```python
from build123d import *

# Parameters (mm, degrees)
SKETCH_1_R          = 3.5
EXTRUDE_1_DEPTH     = 4
SKETCH_3_R          = 3.5
EXTRUDE_2_DEPTH     = 2.9
SKETCH_4_W          = 4.5
SKETCH_4_H          = 4.5
EXTRUDE_3_DEPTH     = 2.5
SKETCH_7_R          = 3.5
CUT_EXTRUDE_1_DEPTH = 10


with BuildPart() as part:
    # 草图1 → 凸台-拉伸1 (new body)
    with BuildSketch(Plane(origin=(0, 0, 0), x_dir=(1, 0, 0), z_dir=(0, 1, 0))):
        Circle(SKETCH_1_R)
        with BuildLine():
            Line((-2.25, 2.25), (-0.4, 2.25))
            ThreePointArc((-0.4, 2.25), (0, 2.65), (0.4, 2.25))
            Line((0.4, 2.25), (2.25, 2.25))
            Line((2.25, 2.25), (2.25, 0.4))
            ThreePointArc((2.25, 0.4), (2.65, 0), (2.25, -0.4))
            Line((2.25, -0.4), (2.25, -2.25))
            Line((2.25, -2.25), (0.4, -2.25))
            ThreePointArc((0.4, -2.25), (0, -2.65), (-0.4, -2.25))
            Line((-0.4, -2.25), (-2.25, -2.25))
            Line((-2.25, -2.25), (-2.25, -0.4))
            ThreePointArc((-2.25, -0.4), (-2.65, 0), (-2.25, 0.4))
            Line((-2.25, 0.4), (-2.25, 2.25))
        make_face(mode=Mode.SUBTRACT)
    extrude(amount=EXTRUDE_1_DEPTH)

    # 草图3 → 凸台-拉伸2 (add)
    with BuildSketch(Plane(origin=(0, 4, 0), x_dir=(1, 0, 0), z_dir=(0, 1, 0))):
        Circle(SKETCH_3_R)
    extrude(amount=EXTRUDE_2_DEPTH)

    # 草图4 → 凸台-拉伸3 (add)
    with BuildSketch(Plane(origin=(0, 6.9, 0), x_dir=(1, 0, 0), z_dir=(0, 1, 0))):
        Rectangle(SKETCH_4_W, SKETCH_4_H)
    extrude(amount=EXTRUDE_3_DEPTH)

    # 草图5 → 旋转1 (revolve)
    with BuildSketch(Plane(origin=(0, 9.4, 0), x_dir=(1, 0, 0), z_dir=(0, 1, 0))):
        with BuildLine():
            Line((-2.75, 0), (-1.75, 0))
            ThreePointArc((-1.75, 0), (-2.25, -0.5), (-2.75, 0))
        make_face()
        with BuildLine():
            Line((1.75, 0), (2.75, 0))
            ThreePointArc((2.75, 0), (2.25, -0.5), (1.75, 0))
        make_face()
    revolve(axis=Axis((-2.75, 9.4, 0), (1, 0, 0)))

    # 草图6 → 旋转2 (revolve)
    with BuildSketch(Plane(origin=(0, 9.4, 0), x_dir=(1, 0, 0), z_dir=(0, 1, 0))):
        with BuildLine():
            Line((0, -2.75), (0, -1.75))
            ThreePointArc((0, -1.75), (-0.5, -2.25), (0, -2.75))
        make_face()
        with BuildLine():
            Line((0, 1.75), (0, 2.75))
            ThreePointArc((0, 2.75), (-0.5, 2.25), (0, 1.75))
        make_face()
    revolve(axis=Axis((0, 9.4, 2.75), (0, 0, -1)))

    # 草图7 → 切除-拉伸1 (cut)
    with BuildSketch(Plane(origin=(0, 9.4, 0), x_dir=(1, 0, 0), z_dir=(0, 1, 0))):
        Circle(SKETCH_7_R)
    extrude(amount=CUT_EXTRUDE_1_DEPTH, mode=Mode.SUBTRACT)


solid = part.part
```
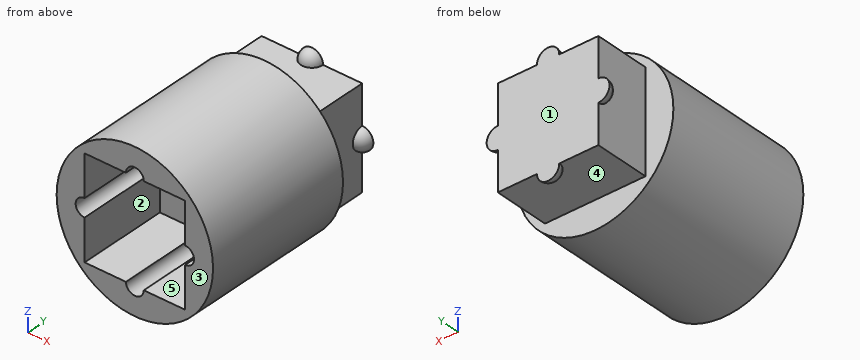
Verification items for the finished model (mm, model axes). Face numbers are marked on the shaded views. A direction names the side the tool comes from. Give positions to 0.01 mm unless a question says otherwise; leave off trailing zeros. Loops run counter-clockwise (first coordinate to the right, second up) from the corner with the lowest first, then second, coordinate; pieces in that order, holes last. Notation, with made-up numbers: M 56,38 L 110,38 A38 cw 110,77 Z; hole C 6,36 d10. An arc over 180 degrees is marked long. Return JSON: item names as keys, results as strings.
1) Gauge pin test, flat ends, axial feed: P1, Ø1, axis at y = 8, z = -1.5, coming from the +X side; P2, Ø1.5, axis at y = 2, z = 1, coming from the +X side; P3, Ø0.6, axis at y = 2.5, z = -1, coming from the -X side. Record the tip position at first contact, or that the pin passes through.
Findings:
{"P1": "stops at x = 2.25", "P2": "stops at x = 3.49", "P3": "stops at x = -3.43"}
2) Section check C-C, the plane x = 0. Enter the section's corners in (y, z).
Findings:
{"outline": "M 0,-3.5 L 6.9,-3.5 L 6.9,-2.25 L 8.9,-2.25 A0.5 ccw 9.4,-2.75 L 9.4,2.75 A0.5 ccw 8.9,2.25 L 6.9,2.25 L 6.9,3.5 L 0,3.5 L 0,2.65 L 4,2.65 L 4,-2.65 L 0,-2.65 Z"}
3) Section check D-D, the plane y = 8. Enter the section's corners in (x, z), and give its area (4 significant figures).
Findings:
{"outline": "M -2.25,-2.25 L 2.25,-2.25 L 2.25,2.25 L -2.25,2.25 Z", "area": "20.25 mm2"}
4) Mould release check, pull along Y, two halves, no side actions. Record for the marked faces 3, 4 and 5: released by +Y, released by -Y, zero draft, split by the parting line, or undercut.
Findings:
{"face 3": "released by -Y", "face 4": "undercut", "face 5": "zero draft"}
5) Tool access check on the marked faces 1 and 2. Record the directions out of +Z, -Z, +X, -X, +Y, -Y that give a thin tool (end or side, any length) a straight path to the whole face; none if there is none.
Findings:
{"face 1": "+Z, -Z, +X, -X, +Y", "face 2": "-Y"}
6) Material ranges on L1, parallel to Y at x = 1.25, z = 1; L2, parallel to Z at x = -1.25, y = 7.5; L3, parallel to X at y = 1.5, z = 1.25, recorded low to high. Write a range as [from, to].
Findings:
{"L1": "y = [4, 9.4]", "L2": "z = [-2.25, 2.25]", "L3": "x = [-3.27, -2.25], [2.25, 3.27]"}
7) Section check A-A, the plane y = 1.25. Enter the section's corners in (x, z), and give its area (3 significant figures).
Findings:
{"outline": "C 0,0 d7; hole M -2.25,-2.25 L -0.4,-2.25 A0.4 ccw 0.4,-2.25 L 2.25,-2.25 L 2.25,-0.4 A0.4 ccw 2.25,0.4 L 2.25,2.25 L 0.4,2.25 A0.4 ccw -0.4,2.25 L -2.25,2.25 L -2.25,0.4 A0.4 ccw -2.25,-0.4 Z", "area": "17.2 mm2"}
8) Section check B-B, the plane z = 0. Enter the section's corners in (x, y), and give its area (3 significant figures).
Findings:
{"outline": "M -3.5,0 L -2.65,0 L -2.65,4 L 2.65,4 L 2.65,0 L 3.5,0 L 3.5,6.9 L 2.25,6.9 L 2.25,8.9 A0.5 ccw 2.75,9.4 L -2.75,9.4 A0.5 ccw -2.25,8.9 L -2.25,6.9 L -3.5,6.9 Z", "area": "38.7 mm2"}
